```python
from build123d import *

# Parameters (mm, degrees)
CYLINDER019_R     = 1
CYLINDER019_DEPTH = 10
ARRAY022_X_COUNT  = 2
ARRAY022_X_PITCH  = 4
ARRAY022_Z_COUNT  = 2
ARRAY022_Z_PITCH  = 4
CYLINDER018_R     = 0.875
CYLINDER018_DEPTH = 10
ARRAY020_Z_COUNT  = 5
ARRAY020_Z_PITCH  = 2.5
BOX014_W          = 8
BOX014_H          = 2
BOX014_DEPTH      = 25


with BuildPart() as cameramountplaneconnectorscrews:
    # Cylinder019 → Cylinder019 (new body)
    with BuildSketch(Plane(origin=(2, 5, 19), x_dir=(1, 0, 0), z_dir=(0, -1, 0))):
        Circle(CYLINDER019_R)
    extrude(amount=CYLINDER019_DEPTH)

    # Array022 X: CameraMountPlaneConnectorScrews ×2


with BuildPart() as cameramountplaneconnectorscrews_1:
    add(cameramountplaneconnectorscrews.part)
    with Locations(*[(-i * ARRAY022_X_PITCH, 0, 0) for i in range(1, ARRAY022_X_COUNT)]):
        add(cameramountplaneconnectorscrews.part)

    # Array022 Z: CameraMountPlaneConnectorScrews ×2


with BuildPart() as cameramountplaneconnectorscrews_2:
    add(cameramountplaneconnectorscrews_1.part)
    with Locations(*[(0, 0, i * ARRAY022_Z_PITCH) for i in range(1, ARRAY022_Z_COUNT)]):
        add(cameramountplaneconnectorscrews_1.part)


with BuildPart() as servoscrewcutters:
    # Cylinder018 → Cylinder018 (new body)
    with BuildSketch(Plane(origin=(0, 5, 0.875), x_dir=(1, 0, 0), z_dir=(0, -1, 0))):
        Circle(CYLINDER018_R)
    extrude(amount=CYLINDER018_DEPTH)

    # Array020 Z: ServoScrewCutters ×5


with BuildPart() as servoscrewcutters_1:
    add(servoscrewcutters.part)
    with Locations(*[(0, 0, i * ARRAY020_Z_PITCH) for i in range(1, ARRAY020_Z_COUNT)]):
        add(servoscrewcutters.part)


with BuildPart() as obj1:
    # Box014 → Box014 (new body)
    with BuildSketch(Plane(origin=(-4, -1, 0), x_dir=(1, 0, 0), z_dir=(0, 0, 1))):
        with Locations((4, 1)):
            Rectangle(BOX014_W, BOX014_H)
    extrude(amount=BOX014_DEPTH)

    # Cut040: cut ServoScrewCutters
    add(servoscrewcutters_1.part, mode=Mode.SUBTRACT)

    # Cut041: cut CameraMountPlaneConnectorScrews
    add(cameramountplaneconnectorscrews_2.part, mode=Mode.SUBTRACT)


solid = obj1.part
```
Verification items for the finished model (mm, model axes). Coordinates: 2 decimals unless noted, no trailing zeros. Write each loop counter-clockwise with the first axis right and the second up, starting at its lowest first coordinate (ties: lowest second). Pieces come first, ordered by that corner, then holes. Notation, with made-up numbers: (1.5, -2.75) - (22.5, -2.75) arc R21 cw to (22.5, 5.25) - close; hole circle Ø8 at (39, 38.25). An arc over 180 degrees is marked (long way). Write item = value, one per line.
Q1. Cross-section at A-A (x = 2). Enter the section's corners in (y, z).
Answer:
outline = (-1, 0) - (1, 0) - (1, 18) - (-1, 18) - close; (-1, 20) - (1, 20) - (1, 22) - (-1, 22) - close; (-1, 24) - (1, 24) - (1, 25) - (-1, 25) - close
Q2. Mould release check, pull along Z, two halves, no side actions. Record for faces 1 (the face through (-0.114, 0.014, 9.243)), 2 (the face through (2, 0, 0)), 3 (the face through (0, 1, 12)): released by +Z, released by -Z, zero draft, split by the parting line, or undercut.
Answer:
face_1 = undercut
face_2 = released by -Z
face_3 = zero draft
Q3. Cross-section at B-B (z = 19). Enter the section's corners in (x, y), plus the area to 3 significant figures.
Answer:
outline = (-4, -1) - (-3, -1) - (-3, 1) - (-4, 1) - close; (-1, -1) - (1, -1) - (1, 1) - (-1, 1) - close; (3, -1) - (4, -1) - (4, 1) - (3, 1) - close
area = 8.00 mm²
Q4. Cross-section at C-C (z = 3.75). Enter the section's corners in (x, y), plus the area to 3 significant figures.
Answer:
outline = (-4, -1) - (-0.79, -1) - (-0.79, 1) - (-4, 1) - close; (0.79, -1) - (4, -1) - (4, 1) - (0.79, 1) - close
area = 12.8 mm²
Q5. Go/stop test with a flat-tipped pin: pin 1 Ø1.8 at (x, z) = (-2, 23) entering from +Y. Record where the tip stops, or that it passes through.
Answer:
pin_1 = through
Q6. Material ranges on L1, parallel to X at y = -0.2, z = 23; L2, parallel to Z at x = 2, y = 0.2; L3, parallel to Z at x = -2.75, y = 0.1, recorded low to high. Write a range as from..to.
Answer:
L1 = -4..-3, -1..1, 3..4
L2 = 0..18, 20..22, 24..25
L3 = 0..18.34, 19.66..22.34, 23.66..25
